Autodesk Inventor part; units mm, degrees
ref_plane "YZ Plane" through (0, 0, 0) normal (1, 0, 0) x (0, 1, 0)
ref_plane "XZ Plane" through (0, 0, 0) normal (0, 1, 0) x (-1, 0, 0)
ref_plane "XY Plane" through (0, 0, 0) normal (0, 0, 1) x (1, 0, 0)
sketch "Sketch1" plane through (0, 0, 0) normal (0, 0, 1) x (1, 0, 0)
  line L0 (0, 0) -> (25.4, 0)
  line L1 (25.4, 0) -> (25.4, 101.6)
  line L2 (25.4, 101.6) -> (0, 101.6)
  line L3 (0, 101.6) -> (0, 0)
  line L4 (12.7, 0) -> (12.7, 12.7) construction
  line L5 (12.7, 101.6) -> (12.7, 88.9) construction
  circle A0 centre (12.7, 12.7) radius 2.5797
  line L6 (12.7, 88.9) -> (12.7, 63.5) construction
  line L7 (10.1203, 88.9) -> (10.1203, 63.5)
  line L8 (15.2797, 63.5) -> (15.2797, 88.9)
  arc A1 (15.2797, 88.9) -> (10.1203, 88.9) centre (12.7, 88.9) ccw
  arc A2 (10.1203, 63.5) -> (15.2797, 63.5) centre (12.7, 63.5) ccw
  point P0 (12.7, 76.2)
  dimension "d0" = 25.4
  dimension "d1" = 101.6
  dimension "d2" = 12.7
  dimension "d3" = 12.7
  dimension "d7" = 25.4
extrude "Extrusion2" add sketch "Sketch1" along normal blind 3.175
properties part number "Slot Bumper attachment"
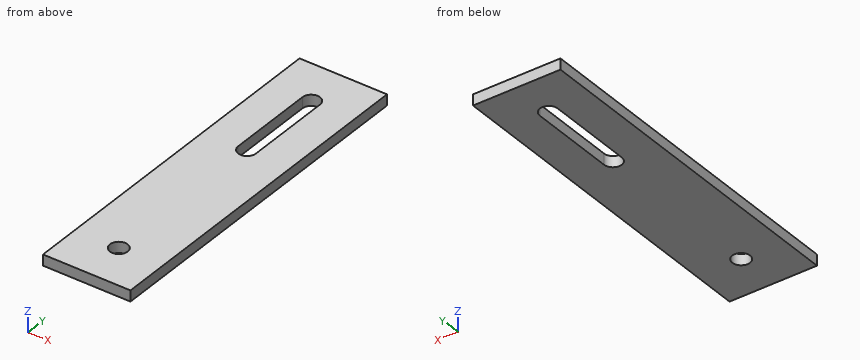
Build history of the part. All positions in model axes, mm. Give positions to 0.01 mm unless a question says otherwise; leave off trailing zeros. Loops run counter-clockwise (first coordinate to the right, second up) from the corner with the lowest first, then second, coordinate; pieces in that order, holes last. Notation, with made-up numbers: (34.25, -10) - (64.25, -10) arc R15 cw to (64.25, 7) - close; hole circle Ø10 at (-22, -0.75). An arc over 180 degrees is marked (long way). Write item = value, one per line. Start each with the question number.
1) Probe probe 1 along Y at (x, z) = (12.7, 0.9); probe 2 along X at (y, z) = (74.5, 1.3); probe 3 along Y at (x, z) = (14.25, 2.3). List the from-to ranges inside material, lowest first. Write a range as from..to.
2) Band-saw the part on A-A on z = 2.15. Give the cut face in (x, y).
3) Band-saw the part on C-C on y = 78.5. Give the cut face in (x, z) (3 decimals).
4) Drop a flat-ended pin along its axis: pin 1 Ø6.5 at (x, y) = (12.7, 12.7) entering from +Z (3 decimals). Give the stop position or say it passes through.
5) Band-saw the part on B-B on x = 12.7. Give the cut face in (y, z) (3 decimals), plus the area to 3 significant figures.
Final values:
q1.probe_1 = 0..10.12, 15.28..60.92, 91.48..101.6
q1.probe_2 = 0..10.12, 15.28..25.4
q1.probe_3 = 0..10.64, 14.76..61.44, 90.96..101.6
q2.outline = (0, 0) - (25.4, 0) - (25.4, 101.6) - (0, 101.6) - close; hole circle Ø5.16 at (12.7, 12.7); hole (10.12, 63.5) arc R2.58 ccw to (15.28, 63.5) - (15.28, 88.9) arc R2.58 ccw to (10.12, 88.9) - close
q3.outline = (0, 0) - (10.12, 0) - (10.12, 3.175) - (0, 3.175) - close; (15.28, 0) - (25.4, 0) - (25.4, 3.175) - (15.28, 3.175) - close
q4.pin_1 = 3.175
q5.outline = (0, 0) - (10.12, 0) - (10.12, 3.175) - (0, 3.175) - close; (15.28, 0) - (60.92, 0) - (60.92, 3.175) - (15.28, 3.175) - close; (91.48, 0) - (101.6, 0) - (101.6, 3.175) - (91.48, 3.175) - close
q5.area = 209 mm²
